For this review, take the finished solid that the model builds, in its own axes (mm). A direction names the side the tool comes from. Give positions to 0.01 mm unless a question says otherwise; leave off trailing zeros. Order: outer loops, then holes, each group sorted by start corner. A loop starts at its lowest first (then second) coordinate and runs counter-clockwise, first axis right, second up. Notation, with made-up numbers: (48.5, -18) - (98.5, -18) arc R30 cw to (98.5, 5) - close; hole circle Ø4 at (51.5, -16.5). An arc over 180 degrees is marked (long way). Use a Markdown table: item, result. Add a question column.
1) Mouldability with a two-part tool opening along Z and no side actions: class faces 1 (the face through (2, -3.175, -85)), 2 (the face through (259.06, 0.04, 68.96)), 3 (the face through (-188.95, 0.04, -114.04)) as released by +Z, released by -Z, zero draft, split by the parting line, or undercut.
2) Clearance check with flat-ended pins moving along their axes: P1, Ø3, axis at x = -145, y = 0.5, coming from the +Z side; P2, Ø3, axis at x = -48, y = 1, coming from the +Z side; P3, Ø3, axis at y = -1, z = -7, coming from the -X side; P4, Ø16.5, axis at x = 42.86, z = 101.6, coming from the -Y side (3 decimals). State where each tip first meets the part, or that it passes through.
3) We need section D-D on x = 310. Write out the cut boundary in (y, z) (3 decimals), then the cut area to 3 significant figures.
4) We need section A-A on y = 1. Write out the cut boundary in (x, z), then the cut area to 3 significant figures.
5) Machinability: for faces 4 (the face through (259.46, 0.04, -68.56)), 5 (the face through (394.92, 0.044, -34.035)), which of the approach directions +Z, -Z, +X, -X, +Y, -Y give a long, thin tool a straight path to every point of the face, cutting with its end or side? Answer none if there is none.
6) We need section C-C on x = 104.5. Write out the cut boundary in (y, z) (3 decimals), then the cut area to 3 significant figures.
7) We need section B-B on x = -125. Write out the cut boundary in (y, z) (3 decimals).
8) Wall thickness on L1, parallel to X at y = 3, z = -38.5; L2, parallel to Z at x = -175, y = 1; L3, parallel to X at y = -0.75, z = -27: over which ranges is each line inside the solid? List them lowest first.
```python
from build123d import *

# Parameters (mm, degrees)
BOSS_EXTRUDE1_DEPTH     = 3.175
SKETCH2_R               = 5.159375
CUT_EXTRUDE1_DEPTH      = 4.175
CUT_EXTRUDE1_DEPTH_BACK = 4.175


with BuildPart() as part:
    # Sketch1 → Boss-Extrude1 (new body, symmetric)
    with BuildSketch(Plane(origin=(0, 0, 0), x_dir=(1, 0, 0), z_dir=(0, 1, 0))):
        Polygon((-372.691935385, 67.129264749), (0, 162.283527596), (372.691935385, 67.129264749), (417.779308923, 0), (372.691935385, -67.129264749), (0, -162.283527596), (-372.691935385, -67.129264749), (-417.779308923, 0), align=None)
    extrude(amount=BOSS_EXTRUDE1_DEPTH, both=True)

    # Sketch2 → Cut-Extrude1 (cut, two sides)
    with BuildSketch(Plane(origin=(0, 0, 0), x_dir=(1, 0, 0), z_dir=(0, 1, 0))) as cut_extrude1_sk:
        with Locations((42.8625, 101.6)):
            Circle(SKETCH2_R)
        with Locations((-42.8625, 101.6)):
            Circle(SKETCH2_R)
        with Locations((-42.8625, -101.6)):
            Circle(SKETCH2_R)
        with Locations((42.8625, -101.6)):
            Circle(SKETCH2_R)
        with BuildLine():
            Line((241.3, 76.2), (-241.3, 76.2))
            ThreePointArc((-241.3, 76.2), (-259.260512242, 68.760512242), (-266.7, 50.8))
            Line((-266.7, 50.8), (-266.7, -50.8))
            ThreePointArc((-266.7, -50.8), (-259.260512242, -68.760512242), (-241.3, -76.2))
            Line((-241.3, -76.2), (241.3, -76.2))
            ThreePointArc((241.3, -76.2), (259.260512242, -68.760512242), (266.7, -50.8))
            Line((266.7, -50.8), (266.7, 50.8))
            ThreePointArc((266.7, 50.8), (259.260512242, 68.760512242), (241.3, 76.2))
        make_face()
    extrude(amount=CUT_EXTRUDE1_DEPTH, mode=Mode.SUBTRACT)
    extrude(cut_extrude1_sk.sketch, amount=-CUT_EXTRUDE1_DEPTH_BACK, mode=Mode.SUBTRACT)


solid = part.part
```
Checked values:
| question | item | result |
|---|---|---|
| 1 | face 1 | zero draft |
| 1 | face 2 | undercut |
| 1 | face 3 | released by -Z |
| 2 | P1 | z = 125.65 |
| 2 | P2 | z = 150.41 |
| 2 | P3 | x = -414.09 |
| 2 | P4 | y = -3.175 |
| 3 | outline | (-3.175, -83.136) - (3.175, -83.136) - (3.175, 83.136) - (-3.175, 83.136) - close |
| 3 | area | 1,060 mm² |
| 4 | outline | (-417.78, 0) - (-372.69, -67.13) - (0, -162.28) - (372.69, -67.13) - (417.78, 0) - (372.69, 67.13) - (0, 162.28) - (-372.69, 67.13) - close; hole (-266.7, -50.8) arc R25.4 ccw to (-241.3, -76.2) - (241.3, -76.2) arc R25.4 ccw to (266.7, -50.8) - (266.7, 50.8) arc R25.4 ccw to (241.3, 76.2) - (-241.3, 76.2) arc R25.4 ccw to (-266.7, 50.8) - close; hole circle Ø10.32 at (-42.86, -101.6); hole circle Ø10.32 at (-42.86, 101.6); hole circle Ø10.32 at (42.86, -101.6); hole circle Ø10.32 at (42.86, 101.6) |
| 4 | area | 96,000 mm² |
| 5 | face 4 | +Y, -Y |
| 5 | face 5 | -Z, +X, +Y, -Y |
| 6 | outline | (-3.175, -135.603) - (3.175, -135.603) - (3.175, -76.2) - (-3.175, -76.2) - close; (-3.175, 76.2) - (3.175, 76.2) - (3.175, 135.603) - (-3.175, 135.603) - close |
| 6 | area | 754 mm² |
| 7 | outline | (-3.175, -130.369) - (3.175, -130.369) - (3.175, -76.2) - (-3.175, -76.2) - close; (-3.175, 76.2) - (3.175, 76.2) - (3.175, 130.369) - (-3.175, 130.369) - close |
| 8 | L1 | -391.92 to -266.7, 266.7 to 391.92 |
| 8 | L2 | -117.6 to -76.2, 76.2 to 117.6 |
| 8 | L3 | -399.64 to -266.7, 266.7 to 399.64 |
